from build123d import *

# Parameters (mm, degrees)
SKETCH_W        = 50
SKETCH_H        = 20
PAD_DEPTH       = 10
SKETCH001_W     = 42.5
SKETCH001_H     = 10
POCKET_DEPTH    = 7
SKETCH002_R     = 1.6
POCKET001_DEPTH = 5
POCKET002_DEPTH = 6.9
SKETCH004_R     = 1.6
POCKET003_DEPTH = 10
SKETCH005_W     = 5.7
SKETCH005_H     = 2.6
POCKET004_DEPTH = 6.15
SKETCH006_R     = 1.6
POCKET005_DEPTH = 10


with BuildPart() as part:
    # Sketch → Pad (new body)
    with BuildSketch(Plane.XY):
        with Locations((25, 10)):
            Rectangle(SKETCH_W, SKETCH_H)
    extrude(amount=PAD_DEPTH)

    # Sketch001 (on Face6 of Pad) → Pocket (cut)
    with BuildSketch(Plane.XY.offset(10)):
        with Locations((25, 15)):
            Rectangle(SKETCH001_W, SKETCH001_H)
    extrude(amount=-POCKET_DEPTH, mode=Mode.SUBTRACT)

    # Sketch002 (on Face6 of Pocket) → Pocket001 (cut)
    with BuildSketch(Plane.XY.offset(3)):
        with Locations((9.5, 15.7)):
            Circle(SKETCH002_R)
        with Locations((40.5, 15.7)):
            Circle(SKETCH002_R)
    extrude(amount=-POCKET001_DEPTH, mode=Mode.SUBTRACT)

    # Sketch003 (on Face4 of Pocket001) → Pocket002 (cut)
    with BuildSketch(Plane.XY.offset(10)):
        Polygon((5.1, 0), (7.6, 6.1), (0, 6.1), (0, 0), align=None)
        Polygon((19.9, 0), (17.4, 6.1), (32.6, 6.1), (30.1, 0), align=None)
        Polygon((42.4, 6.1), (44.9, 0), (50, 0), (50, 6.1), align=None)
    extrude(amount=-POCKET002_DEPTH, mode=Mode.SUBTRACT)

    # Sketch004 (on Face4 of Pocket002) → Pocket003 (cut)
    with BuildSketch(Plane.XY.offset(10)):
        with Locations((12.5, 3)):
            Circle(SKETCH004_R)
        with Locations((37.5, 3)):
            Circle(SKETCH004_R)
    extrude(amount=-POCKET003_DEPTH, mode=Mode.SUBTRACT)

    # Sketch005 (on Face4 of Pocket003) → Pocket004 (cut)
    with BuildSketch(Plane.XY.offset(10)):
        with Locations((12.5, 3)):
            Rectangle(SKETCH005_W, SKETCH005_H)
        with Locations((37.5, 3)):
            Rectangle(SKETCH005_W, SKETCH005_H)
    extrude(amount=-POCKET004_DEPTH, mode=Mode.SUBTRACT)

    # Sketch006 (on Face9 of Pocket004) → Pocket005 (cut)
    with BuildSketch(Plane.XZ):
        with Locations((12.5, 7)):
            Circle(SKETCH006_R)
        with Locations((37.5, 7)):
            Circle(SKETCH006_R)
    extrude(amount=-POCKET005_DEPTH, mode=Mode.SUBTRACT)


solid = part.part
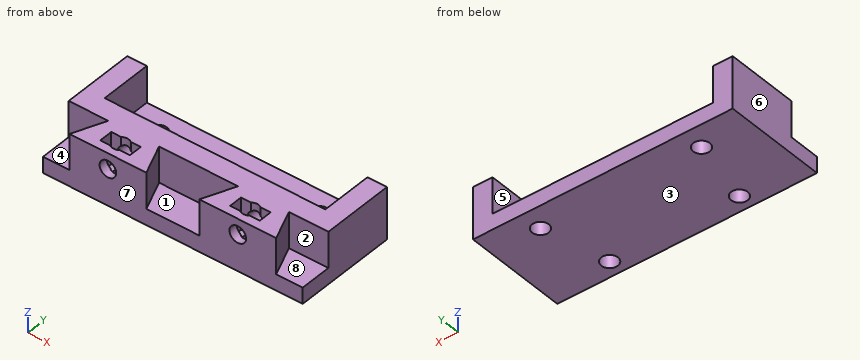
Check sheet for the modelled part. Datum: model origin and axes. Units: mm. Face numbers are marked on the shaded views. A direction names the side the tool comes from. Give positions to 0.01 mm unless a question says otherwise; leave off trailing zeros. Write each loop counter-clockwise with the first axis right and the second up, starting at its lowest first coordinate (ties: lowest second). Pieces come first, ordered by that corner, then holes. Notation, with made-up numbers: (88.25, 2) -> (118.25, 2) arc R16 ccw to (118.25, 26) -> close; hole circle Ø6 at (14, 18.25). An arc over 180 degrees is marked (long way). Use one line per item in the form item = value. Start each with the question number.
1. Access from +Z, -Z, +X, -X, +Y, -Y to the whole of each face (thin tool, end or side, straight path). Record for the marked faces 1, 2, 3, 4 and 5.
2. Thickness scan on line 1 along Y through (x, z) = (37.5, 4.45); line 2 along Y through (x, z) = (14.5, 9); line 3 along X through (y, z) = (15.75, 5.25). Record the ranges inside material, lowest first. Write a range as from..to.
3. Section check D-D (y = 8). Record the cut outline in (x, z), and give its area (3 significant figures).
4. Go/stop test with flat-tipped pins: P1, Ø10, axis at x = 31.5, y = 12.5, coming from the -Z side; P2, Ø3, axis at x = 4.5, y = 3, coming from the +Z side; P3, Ø1, axis at x = 26, z = 8, coming from the +Y side; P4, Ø3, axis at x = 12.5, z = 7, coming from the -Y side. Record where each tip stops, or that it passes through.
5. Section check C-C (x = 12.5). Record the cut outline in (y, z), and give its area (3 significant figures).
6. Mould release check, pull along Y, two halves, no side actions. Record for the marked faces 6, 7 and 8: pulls with the +Y half, pulls with the -Y half, needs draft (parallel to the pull), parting line crosses it, or undercut.
7. Section check B-B (z = 2.5). Record the cut outline in (x, y).
8. Section check A-A (y = 15.7). Record the cut outline in (x, z), and give its area (3 significant figures).
Conclusion:
q1.face_1 = +Z
q1.face_2 = +Z, +X
q1.face_3 = -Z, +X, -X, +Y, -Y
q1.face_4 = +Z, -X
q1.face_5 = +Z, +Y
q2.line_1 = 0..1.4, 4.6..10
q2.line_2 = 0..1.7, 4.3..10
q2.line_3 = 0..3.75, 46.25..50
q3.outline = (0, 0) -> (50, 0) -> (50, 10) -> (0, 10) -> close; hole circle Ø3.2 at (12.5, 7); hole circle Ø3.2 at (37.5, 7)
q3.area = 484 mm²
q4.P1 = 0
q4.P2 = 3.1
q4.P3 = 10
q4.P4 = through
q5.outline = (0, 0) -> (1.4, 0) -> (1.4, 5.4) -> (0, 5.4) -> close; (0, 8.6) -> (1.4, 8.6) -> (1.4, 10) -> (0, 10) -> close; (4.6, 0) -> (20, 0) -> (20, 3) -> (10, 3) -> (10, 5.4) -> (4.6, 5.4) -> close; (4.6, 8.6) -> (10, 8.6) -> (10, 10) -> (4.6, 10) -> close
q5.area = 76.2 mm²
q6.face_6 = needs draft
q6.face_7 = pulls with the -Y half
q6.face_8 = undercut
q7.outline = (0, 0) -> (50, 0) -> (50, 20) -> (0, 20) -> close; hole circle Ø3.2 at (9.5, 15.7); hole circle Ø3.2 at (12.5, 3); hole circle Ø3.2 at (37.5, 3); hole circle Ø3.2 at (40.5, 15.7)
q8.outline = (0, 0) -> (7.9, 0) -> (7.9, 3) -> (3.75, 3) -> (3.75, 10) -> (0, 10) -> close; (11.1, 0) -> (38.9, 0) -> (38.9, 3) -> (11.1, 3) -> close; (42.1, 0) -> (50, 0) -> (50, 10) -> (46.25, 10) -> (46.25, 3) -> (42.1, 3) -> close
q8.area = 183 mm²
